Here's how the part is built. I have some questions about the finished solid (model axes, mm). A direction names the side the tool comes from. Round coordinates to 2 decimals unless told otherwise and drop trailing zeros. Order: outer loops, then holes, each group sorted by start corner. A loop starts at its lowest first (then second) coordinate and runs counter-clockwise, first axis right, second up. Notation, with made-up numbers: (78, 2) -> (90, 2) arc R13 cw to (90, 20) -> close; hole circle Ø2 at (43, 53.5). An arc over 180 degrees is marked (long way). One line per item, written item: value.
```python
from build123d import *

# Parameters (mm, degrees)
SKETCH_1_R      = 40
SKETCH_1_R_2    = 2
SKETCH_1_R_3    = 3
SKETCH_1_R_4    = 1.5
EXTRUDE_1_DEPTH = 2


with BuildPart() as part:
    # 草图1 → 凸台-拉伸1 (new body)
    with BuildSketch(Plane(origin=(0, 0, 0), x_dir=(1, 0, 0), z_dir=(0, 1, 0))):
        with Locations(Location((0, 0, 0), (0, 0, 270))):
            Circle(SKETCH_1_R)
        with Locations(Location((-24.395, 24.395, 0), (0, 0, 270))):
            Circle(SKETCH_1_R_2, mode=Mode.SUBTRACT)
        with Locations(Location((24.395, 24.395, 0), (0, 0, 270))):
            Circle(SKETCH_1_R_2, mode=Mode.SUBTRACT)
        with Locations(Location((24.395, -24.395, 0), (0, 0, 270))):
            Circle(SKETCH_1_R_2, mode=Mode.SUBTRACT)
        with Locations(Location((-24.395, -24.395, 0), (0, 0, 270))):
            Circle(SKETCH_1_R_2, mode=Mode.SUBTRACT)
        with Locations(Location((0, -30, 0), (0, 0, 270))):
            Circle(SKETCH_1_R_3, mode=Mode.SUBTRACT)
        with Locations(Location((0, -23, 0), (0, 0, 270))):
            Circle(SKETCH_1_R_4, mode=Mode.SUBTRACT)
        with Locations(Location((4.949747468, -25.050252532, 0), (0, 0, 270))):
            Circle(SKETCH_1_R_4, mode=Mode.SUBTRACT)
        with Locations(Location((7, -30, 0), (0, 0, 270))):
            Circle(SKETCH_1_R_4, mode=Mode.SUBTRACT)
        with Locations(Location((4.949747468, -34.949747468, 0), (0, 0, 270))):
            Circle(SKETCH_1_R_4, mode=Mode.SUBTRACT)
        with Locations(Location((0, -37, 0), (0, 0, 270))):
            Circle(SKETCH_1_R_4, mode=Mode.SUBTRACT)
        with Locations(Location((-4.949747468, -34.949747468, 0), (0, 0, 270))):
            Circle(SKETCH_1_R_4, mode=Mode.SUBTRACT)
        with Locations(Location((-7, -30, 0), (0, 0, 270))):
            Circle(SKETCH_1_R_4, mode=Mode.SUBTRACT)
        with Locations(Location((-4.949747468, -25.050252532, 0), (0, 0, 270))):
            Circle(SKETCH_1_R_4, mode=Mode.SUBTRACT)
        with Locations(Location((0, 30, 0), (0, 0, 270))):
            Circle(SKETCH_1_R_3, mode=Mode.SUBTRACT)
        with Locations(Location((4.949747468, 25.050252532, 0), (0, 0, 270))):
            Circle(SKETCH_1_R_4, mode=Mode.SUBTRACT)
        with Locations(Location((7, 30, 0), (0, 0, 270))):
            Circle(SKETCH_1_R_4, mode=Mode.SUBTRACT)
        with Locations(Location((4.949747468, 34.949747468, 0), (0, 0, 270))):
            Circle(SKETCH_1_R_4, mode=Mode.SUBTRACT)
        with Locations(Location((0, 37, 0), (0, 0, 270))):
            Circle(SKETCH_1_R_4, mode=Mode.SUBTRACT)
        with Locations(Location((-4.949747468, 34.949747468, 0), (0, 0, 270))):
            Circle(SKETCH_1_R_4, mode=Mode.SUBTRACT)
        with Locations(Location((-7, 30, 0), (0, 0, 270))):
            Circle(SKETCH_1_R_4, mode=Mode.SUBTRACT)
        with Locations(Location((-4.949747468, 25.050252532, 0), (0, 0, 270))):
            Circle(SKETCH_1_R_4, mode=Mode.SUBTRACT)
        with Locations(Location((0, 23, 0), (0, 0, 270))):
            Circle(SKETCH_1_R_4, mode=Mode.SUBTRACT)
        with Locations(Location((-30, 0, 0), (0, 0, 270))):
            Circle(SKETCH_1_R_3, mode=Mode.SUBTRACT)
        with Locations(Location((-23, 0, 0), (0, 0, 270))):
            Circle(SKETCH_1_R_4, mode=Mode.SUBTRACT)
        with Locations(Location((-25.050252532, -4.949747468, 0), (0, 0, 270))):
            Circle(SKETCH_1_R_4, mode=Mode.SUBTRACT)
        with Locations(Location((-30, -7, 0), (0, 0, 270))):
            Circle(SKETCH_1_R_4, mode=Mode.SUBTRACT)
        with Locations(Location((-34.949747468, -4.949747468, 0), (0, 0, 270))):
            Circle(SKETCH_1_R_4, mode=Mode.SUBTRACT)
        with Locations(Location((-37, 0, 0), (0, 0, 270))):
            Circle(SKETCH_1_R_4, mode=Mode.SUBTRACT)
        with Locations(Location((-34.949747468, 4.949747468, 0), (0, 0, 270))):
            Circle(SKETCH_1_R_4, mode=Mode.SUBTRACT)
        with Locations(Location((-30, 7, 0), (0, 0, 270))):
            Circle(SKETCH_1_R_4, mode=Mode.SUBTRACT)
        with Locations(Location((-25.050252532, 4.949747468, 0), (0, 0, 270))):
            Circle(SKETCH_1_R_4, mode=Mode.SUBTRACT)
        with Locations(Location((-15, -5, 0), (0, 0, 270))):
            Circle(SKETCH_1_R_2, mode=Mode.SUBTRACT)
        with Locations(Location((33.5, -5, 0), (0, 0, 270))):
            Circle(SKETCH_1_R_2, mode=Mode.SUBTRACT)
        with Locations(Location((33.5, 5, 0), (0, 0, 270))):
            Circle(SKETCH_1_R_2, mode=Mode.SUBTRACT)
        with Locations(Location((-15, 5, 0), (0, 0, 270))):
            Circle(SKETCH_1_R_2, mode=Mode.SUBTRACT)
        Polygon((-11, -1), (-11, -10.5), (29.5, -10.5), (29.5, -1), (35.5, -1), (35.5, 1), (29.5, 1), (29.5, 10.5), (-11, 10.5), (-11, 1), (-17, 1), (-17, -1), align=None, mode=Mode.SUBTRACT)
    extrude(amount=EXTRUDE_1_DEPTH)


solid = part.part
```
Q1. I need wall thicknesses on line 1 along X through (y, z) = (0.85, 30); line 2 along X through (y, z) = (0.9, -2); line 3 along X through (y, z) = (0.95, 0). Which ranges of each line are inside material? Lowest first, please.
Answers:
line 1: -26.46 to -8.5, -5.5 to -3, 3 to 5.5, 8.5 to 26.46
line 2: -39.95 to -32.24, -27.76 to -11, 29.5 to 39.95
line 3: -40 to -38.5, -35.5 to -33, -27 to -24.5, -21.5 to -17, 35.5 to 40
Q2. For P1, Ø0.6, axis at x = 15.5, y = 1, coming from the -Z side; P2, Ø1, axis at y = 1, z = 6, coming from the +X side; P3, Ø1, axis at x = 14.5, y = 1, coming from the +Z side, each with a flat end and sliding along its axis, tell me the tip position at first contact or that it passes through.
Answers:
P1: z = -37
P2: x = 39.62
P3: z = 37.47
Q3. I want a section at A-A on x = 0. Give the number of separate pieces and of enclosed holes in the cut face, then the cut area to 3 significant figures.
Answers:
separate pieces: 8
enclosed holes: 0
area: 70.0 mm2
Q4. I want a section at D-D on x = -12. Write out the boundary of the cut face in (y, z), then the cut area to 3 significant figures.
Answers:
outline: (0, -38.16) -> (2, -38.16) -> (2, -1) -> (0, -1) -> close; (0, 1) -> (2, 1) -> (2, 38.16) -> (0, 38.16) -> close
area: 149 mm2
Q5. I want a section at C-C on z = 30. Write out the boundary of the cut face in (x, y).
Answers:
outline: (-26.46, 0) -> (-8.5, 0) -> (-8.5, 2) -> (-26.46, 2) -> close; (-5.5, 0) -> (-3, 0) -> (-3, 2) -> (-5.5, 2) -> close; (3, 0) -> (5.5, 0) -> (5.5, 2) -> (3, 2) -> close; (8.5, 0) -> (26.46, 0) -> (26.46, 2) -> (8.5, 2) -> close
Q6. I want a section at B-B on x = -30. Write out the boundary of the cut face in (y, z), then the cut area to 3 significant figures.
Answers:
outline: (0, -26.46) -> (2, -26.46) -> (2, -8.5) -> (0, -8.5) -> close; (0, -5.5) -> (2, -5.5) -> (2, -3) -> (0, -3) -> close; (0, 3) -> (2, 3) -> (2, 5.5) -> (0, 5.5) -> close; (0, 8.5) -> (2, 8.5) -> (2, 26.46) -> (0, 26.46) -> close
area: 81.8 mm2
Q7. Which directions (+Z, -Z, +X, -X, +Y, -Y) give clear straight access to the entire face, cutting with the end or side of a thin tool? Please do faces 1 (the face through (29.5, 1, -6)), 2 (the face through (-17.2, 2, -0.6)).
Answers:
face 1: +Y, -Y
face 2: +Z, -Z, +X, -X, +Y
